```python
from build123d import *

# Parameters (mm, degrees)
F5_W         = 192.786
F5_H         = 141.3764
F7_DEPTH     = 44.45
F12_W        = 187.452
F12_H        = 127
F14_DEPTH    = 38.1
F4_R         = 15.621
F4_R_2       = 13.081
F13_W        = 2.032
F13_H        = 10.16
F13_W_2      = 10.16
F13_H_2      = 2.032
F15_DEPTH    = 8.89
F16_DEPTH    = 2.9972
F17_DEPTH    = 3.81
F10_R        = 2.3749
F18_DEPTH    = 25.4
F3_R         = 1.9304
F19_DEPTH    = 25.4
F11_R        = 2.54
F11_R_2      = 2.794
F20_DEPTH    = 8.89
F21_W        = 8.89
F21_H        = 5.842
F21_W_2      = 9.525
F21_H_2      = 15.621
F22_DEPTH    = 25.4
F23_R        = 2.0828
F24_DEPTH    = 4.318
F25_T1_DEPTH = 41.91
F25_T3_DEPTH = 52.07
F25_T5_DEPTH = 6.35


# Not quite as in the source:
# - a fillet or chamfer that OpenCascade refuses, or shapes differently, is made with other operations: its cross-section is extruded or revolved along the edge and cut away or added


with BuildPart() as f7:
    # F5 (on Top) → F7 (new body)
    with BuildSketch(Plane.XY):
        with Locations((-4.773771323, -23.1295908162)):
            Rectangle(F5_W, F5_H)
    extrude(amount=F7_DEPTH)

    # F12 (on face) → F14 (cut)
    with BuildSketch(Plane.XY.offset(44.45)):
        with Locations((-5.154771323, -23.1295908162)):
            Rectangle(F12_W, F12_H)
    extrude(amount=-F14_DEPTH, mode=Mode.SUBTRACT)

    # F4 (on Top) + F13 (on Top) → F15 (join)
    with BuildSketch(Plane.XY):
        with Locations((-81.989771323, -34.1785908162)):
            Circle(F4_R)
        with Locations((-81.989771323, -34.1785908162)):
            Circle(F4_R_2, mode=Mode.SUBTRACT)
    with BuildSketch(Plane.XY):
        with Locations((18.975228677, 35.2904091838)):
            Rectangle(F13_W, F13_H)
        with Locations((47.6495291469, -25.7965908162)):
            Rectangle(F13_W_2, F13_H_2)
    extrude(amount=F15_DEPTH)

    # F6 (on face) → F16 (cut)
    with BuildSketch(Plane.XY):
        Polygon((-81.6243755079, 34.3379091838), (-79.6079796927, 37.8304091838), (-81.6243755079, 41.3229091838), (-85.6571671382, 41.3229091838), (-87.6735629533, 37.8304091838), (-85.6571671382, 34.3379091838), align=None)
        Polygon((-6.6943755079, 34.3379091838), (-4.6779796927, 37.8304091838), (-6.6943755079, 41.3229091838), (-10.7271671382, 41.3229091838), (-12.7435629533, 37.8304091838), (-10.7271671382, 34.3379091838), align=None)
        Polygon((-30.8243755079, 19.0979091838), (-28.8079796927, 22.5904091838), (-30.8243755079, 26.0829091838), (-34.8571671382, 26.0829091838), (-36.8735629533, 22.5904091838), (-34.8571671382, 19.0979091838), align=None)
        Polygon((-82.8943755079, -14.4300908162), (-80.8779796927, -10.9375908162), (-82.8943755079, -7.4450908162), (-86.9271671382, -7.4450908162), (-88.9435629533, -10.9375908162), (-86.9271671382, -14.4300908162), align=None)
        Polygon((-30.8243755079, -9.3500908162), (-28.8079796927, -5.8575908162), (-30.8243755079, -2.3650908162), (-34.8571671382, -2.3650908162), (-36.8735629533, -5.8575908162), (-34.8571671382, -9.3500908162), align=None)
        Polygon((1.1796244921, -14.4300908162), (3.1960203073, -10.9375908162), (1.1796244921, -7.4450908162), (-2.8531671382, -7.4450908162), (-4.8695629533, -10.9375908162), (-2.8531671382, -14.4300908162), align=None)
    extrude(amount=F16_DEPTH, mode=Mode.SUBTRACT)

    # F9 (on Top) → F17 (cut)
    with BuildSketch(Plane.XY):
        Polygon((-55.7338586688, -33.239207965), (-53.0355544507, -28.565607965), (-55.7338586688, -23.892007965), (-61.130467105, -23.892007965), (-63.828771323, -28.565607965), (-61.130467105, -33.239207965), align=None)
        Polygon((-24.9998586688, -81.067407965), (-22.3015544507, -76.393807965), (-24.9998586688, -71.720207965), (-30.396467105, -71.720207965), (-33.094771323, -76.393807965), (-30.396467105, -81.067407965), align=None)
        Polygon((17.1641413312, -71.720207965), (14.4658371131, -71.720207965), (11.767532895, -71.720207965), (9.069228677, -76.393807965), (11.767532895, -81.067407965), (17.1641413312, -81.067407965), (19.8624455493, -76.393807965), align=None)
        Polygon((-10.8715544507, -28.565607965), (-13.5698586688, -23.892007965), (-18.966467105, -23.892007965), (-21.664771323, -28.565607965), (-18.966467105, -33.239207965), (-13.5698586688, -33.239207965), align=None)
    extrude(amount=F17_DEPTH, mode=Mode.SUBTRACT)

    # F10 (on Top) → F18 (cut)
    with BuildSketch(Plane.XY):
        with Locations((-58.4321628869, -28.565607965)):
            Circle(F10_R)
        with Locations((-27.6981628869, -76.393807965)):
            Circle(F10_R)
        with Locations((-16.2681628869, -28.565607965)):
            Circle(F10_R)
        with Locations((14.4658371131, -76.393807965)):
            Circle(F10_R)
    extrude(amount=F18_DEPTH, mode=Mode.SUBTRACT)

    # F3 (on Top) → F19 (cut)
    with BuildSketch(Plane.XY):
        with Locations((-84.910771323, -10.9375908162)):
            Circle(F3_R)
        with Locations((-32.840771323, -5.8575908162)):
            Circle(F3_R)
        with Locations((-32.840771323, 22.5904091838)):
            Circle(F3_R)
        with Locations((-8.710771323, 37.8304091838)):
            Circle(F3_R)
        with Locations((-83.640771323, 37.8304091838)):
            Circle(F3_R)
        with Locations((-0.836771323, -10.9375908162)):
            Circle(F3_R)
    extrude(amount=F19_DEPTH, mode=Mode.SUBTRACT)

    # F11 (on Top) → F20 (join)
    with BuildSketch(Plane.XY):
        with Locations((-6.1370921321, 28.5807047039)):
            Circle(F11_R)
        with Locations((-51.3140404916, 29.3099723562)):
            Circle(F11_R)
        with Locations((-50.6939233637, -1.3771463051)):
            Circle(F11_R)
        with Locations((-84.7697969953, 15.9851294398)):
            Circle(F11_R_2)
    extrude(amount=F20_DEPTH)

    # F21 (on face) → F22 (cut)
    with BuildSketch(Plane(origin=(-101.166771323, 0, 0), x_dir=(0, -1, 0), z_dir=(-1, 0, 0))):
        with Locations((-12.1256091838, 12.573)):
            Rectangle(F21_W, F21_H)
        with Locations((-28.6356091838, 12.573)):
            Rectangle(F21_W, F21_H)
        with Locations((1.7808908162, 17.4625)):
            Rectangle(F21_W_2, F21_H_2)
    extrude(amount=-F22_DEPTH, mode=Mode.SUBTRACT)

    # F23 (on face) → F24 (cut)
    with BuildSketch(Plane.XY.offset(44.45)):
        with Locations((-96.086771323, -90.2236908162)):
            Circle(F23_R)
        with Locations((86.539228677, -90.2236908162)):
            Circle(F23_R)
        with Locations((86.539228677, 43.9645091838)):
            Circle(F23_R)
        with Locations((-96.086771323, 43.9645091838)):
            Circle(F23_R)
    extrude(amount=-F24_DEPTH, mode=Mode.SUBTRACT)

    # F25: fillet of radius 1.524 on 12 edges, made by hand

    # F25_s2 → F25_t1 (join)
    with BuildSketch(Plane.XY.offset(2.54)):
        with BuildLine():
            ThreePointArc((-97.356771323, -86.6295908162), (-98.4344020576, -86.1832215507), (-98.880771323, -85.1055908162))
            Line((-98.880771323, -85.1055908162), (-98.880771323, -86.6295908162))
            Line((-98.880771323, -86.6295908162), (-97.356771323, -86.6295908162))
        make_face()
        with BuildLine():
            ThreePointArc((88.571228677, -85.1055908162), (88.1248594115, -86.1832215507), (87.047228677, -86.6295908162))
            Line((87.047228677, -86.6295908162), (88.571228677, -86.6295908162))
            Line((88.571228677, -86.6295908162), (88.571228677, -85.1055908162))
        make_face()
    extrude(amount=F25_T1_DEPTH)

    # F25_s4 → F25_t3 (cut)
    with BuildSketch(Plane.XY.offset(-3.81)):
        with BuildLine():
            ThreePointArc((-99.642771323, 47.5586091838), (-100.7204020576, 47.1122399184), (-101.166771323, 46.0346091838))
            Line((-101.166771323, 46.0346091838), (-101.166771323, 47.5586091838))
            Line((-101.166771323, 47.5586091838), (-99.642771323, 47.5586091838))
        make_face()
        with BuildLine():
            ThreePointArc((-101.166771323, -92.2937908162), (-100.7204020576, -93.3714215507), (-99.642771323, -93.8177908162))
            Line((-99.642771323, -93.8177908162), (-101.166771323, -93.8177908162))
            Line((-101.166771323, -93.8177908162), (-101.166771323, -92.2937908162))
        make_face()
        with BuildLine():
            ThreePointArc((91.619228677, -92.2937908162), (91.1728594115, -93.3714215507), (90.095228677, -93.8177908162))
            Line((90.095228677, -93.8177908162), (91.619228677, -93.8177908162))
            Line((91.619228677, -93.8177908162), (91.619228677, -92.2937908162))
        make_face()
        with BuildLine():
            ThreePointArc((90.095228677, 47.5586091838), (91.1728594115, 47.1122399184), (91.619228677, 46.0346091838))
            Line((91.619228677, 46.0346091838), (91.619228677, 47.5586091838))
            Line((91.619228677, 47.5586091838), (90.095228677, 47.5586091838))
        make_face()
    extrude(amount=F25_T3_DEPTH, mode=Mode.SUBTRACT)

    # F25_s6 → F25_t5 (cut)
    with BuildSketch(Plane.XY.offset(6.35)):
        with BuildLine():
            ThreePointArc((17.959228677, 31.7344091838), (18.4055979424, 30.6567784493), (19.483228677, 30.2104091838))
            Line((19.483228677, 30.2104091838), (17.959228677, 30.2104091838))
            Line((17.959228677, 30.2104091838), (17.959228677, 31.7344091838))
        make_face()
        with BuildLine():
            ThreePointArc((42.5695291469, -25.2885908162), (43.0158984124, -26.3662215507), (44.0935291469, -26.8125908162))
            Line((44.0935291469, -26.8125908162), (42.5695291469, -26.8125908162))
            Line((42.5695291469, -26.8125908162), (42.5695291469, -25.2885908162))
        make_face()
        with BuildLine():
            ThreePointArc((42.5695291469, -26.3045908162), (43.0158984124, -25.2269600816), (44.0935291469, -24.7805908162))
            Line((44.0935291469, -24.7805908162), (42.5695291469, -24.7805908162))
            Line((42.5695291469, -24.7805908162), (42.5695291469, -26.3045908162))
        make_face()
        with BuildLine():
            ThreePointArc((19.991228677, 31.7344091838), (19.5448594115, 30.6567784493), (18.467228677, 30.2104091838))
            Line((18.467228677, 30.2104091838), (19.991228677, 30.2104091838))
            Line((19.991228677, 30.2104091838), (19.991228677, 31.7344091838))
        make_face()
        with BuildLine():
            ThreePointArc((51.2055291469, -26.8125908162), (52.2831598814, -26.3662215507), (52.7295291469, -25.2885908162))
            Line((52.7295291469, -25.2885908162), (52.7295291469, -26.8125908162))
            Line((52.7295291469, -26.8125908162), (51.2055291469, -26.8125908162))
        make_face()
        with BuildLine():
            ThreePointArc((51.2055291469, -24.7805908162), (52.2831598814, -25.2269600816), (52.7295291469, -26.3045908162))
            Line((52.7295291469, -26.3045908162), (52.7295291469, -24.7805908162))
            Line((52.7295291469, -24.7805908162), (51.2055291469, -24.7805908162))
        make_face()
    extrude(amount=F25_T5_DEPTH, mode=Mode.SUBTRACT)


solid = f7.part
```
Check sheet for the modelled part. Datum: model origin and axes. Units: mm. A direction names the side the tool comes from. Round coordinates to 2 decimals unless told otherwise and drop trailing zeros. Order: outer loops, then holes, each group sorted by start corner. A loop starts at its lowest first (then second) coordinate and runs counter-clockwise, first axis right, second up.
1) Section check B-B (z = 33.5). Record the boundary of the cut face in (x, y).
2) Section check C-C (y = -52.5). Record the boundary of the cut face in (x, z).
3) Section check D-D (z = 22). Record the boundary of the cut face in (x, y), and give its area (3 significant figures).
4) Mould release check, pull along X, two halves, no side actions. Record for faces 4 (the flat face through (-6, -22, 0)), 5 (the flat face through (-23.63, -74.09, 1.88)): +X half, -X half, draft (parallel to the pull), parting line (faces both ways), or undercut.
5) Section check A-A (z = 12.5). Record the boundary of the cut face in (x, y).
6) Scan lines: line 1 (X direction, y = -30.5, z = 33); line 2 (Y direction, x = -11.5, z = 29); line 3 (Z direction, x = -89.5, y = 33.5). Record each from-to range of solid material in increasing order.
7) Tool access check on faces 1 (the flat face through (-35, 22, 2.997)), 2 (the flat face through (-6, -93.818, 22)), 3 (the cylindrical face through (84.886, 42.697, 42.321)). Record the directions out of +Z, -Z, +X, -X, +Y, -Y that give a thin tool (end or side, any length) a straight path to the whole face; none if there is none.
8) Go/stop test with flat-tipped pins: pin 1 Ø4.5 at (x, y) = (-27.7, -76.39) entering from +Z; pin 2 Ø7.5 at (x, y) = (-58.43, -28.57) entering from -Z; pin 3 Ø3 at (x, y) = (-30.5, 1) entering from +Z; pin 4 Ø5.5 at (x, y) = (-51.5, -1) entering from +Z. Record where each tip stops, or that it passes through.
Result:
1. outline: (-101.17, -92.29) arc R1.52 ccw to (-99.64, -93.82) - (90.1, -93.82) arc R1.52 ccw to (91.62, -92.29) - (91.62, 46.03) arc R1.52 ccw to (90.1, 47.56) - (-99.64, 47.56) arc R1.52 ccw to (-101.17, 46.03) - close; hole (-98.88, -85.11) arc R1.52 ccw to (-97.36, -86.63) - (87.05, -86.63) arc R1.52 ccw to (88.57, -85.11) - (88.57, 40.37) - (-98.88, 40.37) - close
2. outline: (-101.17, 0) - (91.62, 0) - (91.62, 44.45) - (88.57, 44.45) - (88.57, 6.35) - (-98.88, 6.35) - (-98.88, 44.45) - (-101.17, 44.45) - close
3. outline: (-101.17, -92.29) arc R1.52 ccw to (-99.64, -93.82) - (90.1, -93.82) arc R1.52 ccw to (91.62, -92.29) - (91.62, 46.03) arc R1.52 ccw to (90.1, 47.56) - (-99.64, 47.56) arc R1.52 ccw to (-101.17, 46.03) - (-101.17, 2.98) - (-98.88, 2.98) - (-98.88, 40.37) - (88.57, 40.37) - (88.57, -85.11) arc R1.52 cw to (87.05, -86.63) - (-97.36, -86.63) arc R1.52 cw to (-98.88, -85.11) - (-98.88, -6.54) - (-101.17, -6.54) - close
3. area: 3,430 mm2
4. face 4: draft
4. face 5: undercut
5. outline: (-101.17, -92.29) arc R1.52 ccw to (-99.64, -93.82) - (90.1, -93.82) arc R1.52 ccw to (91.62, -92.29) - (91.62, 46.03) arc R1.52 ccw to (90.1, 47.56) - (-99.64, 47.56) arc R1.52 ccw to (-101.17, 46.03) - (-101.17, 33.08) - (-98.88, 33.08) - (-98.88, 40.37) - (88.57, 40.37) - (88.57, -85.11) arc R1.52 cw to (87.05, -86.63) - (-97.36, -86.63) arc R1.52 cw to (-98.88, -85.11) - (-98.88, -6.54) - (-101.17, -6.54) - close; (-101.17, 2.98) - (-98.88, 2.98) - (-98.88, 7.68) - (-101.17, 7.68) - close; (-101.17, 16.57) - (-98.88, 16.57) - (-98.88, 24.19) - (-101.17, 24.19) - close
6. line 1: x = -101.17 to -98.88, 88.57 to 91.62
6. line 2: y = -93.82 to -86.63, 40.37 to 47.56
6. line 3: z = 0 to 6.35
7. face 1: -Z
7. face 2: +Z, -Z, +X, -X, -Y
7. face 3: +Z
8. pin 1: passes through
8. pin 2: stops at z = 3.81
8. pin 3: stops at z = 6.35
8. pin 4: stops at z = 8.89
